```python
from build123d import *

# Parameters (mm, degrees)
F0_W      = 59
F0_H      = 54
F1_DEPTH  = 5
F2_W      = 5
F2_H      = 54
F3_DEPTH  = 21.25
F4_W      = 42
F4_H      = 42
F5_DEPTH  = 9.75
F7_DEPTH  = 33
F8_R      = 1.6
F8_R_2    = 11.5
F9_DEPTH  = 14.751
F10_R     = 2.1
F11_DEPTH = 5.001
F12_SIZE  = 3
F13_R     = 5
F14_R     = 1.6
F15_DEPTH = 2.5
F16_R     = 2.1
F17_DEPTH = 59.001
F19_DEPTH = 10.6937211186


with BuildPart() as f1:
    # F0 (on Top) → F1 (new body)
    with BuildSketch(Plane.XY):
        with Locations((29.5, 27)):
            Rectangle(F0_W, F0_H)
    extrude(amount=F1_DEPTH)

    # F2 (on face) → F3 (join)
    with BuildSketch(Plane.XY.offset(5)):
        with Locations((2.5, 27)):
            Rectangle(F2_W, F2_H)
    extrude(amount=F3_DEPTH)

    # F4 (on face) → F5 (join)
    with BuildSketch(Plane.XY.offset(5)):
        with Locations((38, 21)):
            Rectangle(F4_W, F4_H)
    extrude(amount=F5_DEPTH)

    # F6 (on face) → F7 (cut)
    with BuildSketch(Plane.YZ.offset(59)):
        Polygon((0, 6.5), (0, 0), (33, 0), (19, 6.5), align=None)
    extrude(amount=-F7_DEPTH, mode=Mode.SUBTRACT)

    # F8 (on face) → F9 (cut, through all)
    with BuildSketch(Plane.XY.offset(14.75)):
        with Locations((22.8, 36.2)):
            Circle(F8_R)
        with Locations((38, 21)):
            Circle(F8_R_2)
        with Locations((53.2, 36.2)):
            Circle(F8_R)
        with Locations((22.8, 5.8)):
            Circle(F8_R)
        with Locations((53.2, 5.8)):
            Circle(F8_R)
        with Locations((29.8, 5.8)):
            Circle(F8_R)
    extrude(amount=-F9_DEPTH, mode=Mode.SUBTRACT)

    # F10 (on face) → F11 (cut, through all)
    with BuildSketch(Plane.XY.offset(5)):
        with Locations((37, 48)):
            Circle(F10_R)
        with Locations((51.5, 48)):
            Circle(F10_R)
    extrude(amount=-F11_DEPTH, mode=Mode.SUBTRACT)

    # F12
    f12_edges = [f1.edges().sort_by_distance(p)[0] for p in [
        (59, 54, 2.5),
        (59, 42, 9.875),
        (59, 0, 10.625),
    ]]
    chamfer(f12_edges, length=F12_SIZE)

    # F13
    f13_edges = [f1.edges().sort_by_distance(p)[0] for p in [
        (0, 27, 0),
    ]]
    fillet(f13_edges, radius=F13_R)

    # F14 (on face) → F15 (cut)
    with BuildSketch(Plane.XY.offset(14.75)):
        Polygon((31.417729554, 3.0006632601), (33.0331615075, 5.8013265202), (31.4154319535, 8.6006632601), (28.182270446, 8.5993367399), (26.5668384925, 5.7986734798), (28.1845680465, 2.9993367399), align=None)
        with Locations((29.8, 5.8)):
            Circle(F14_R, mode=Mode.SUBTRACT)
    extrude(amount=-F15_DEPTH, mode=Mode.SUBTRACT)

    # F16 (on face) → F17 (cut, through all)
    with BuildSketch(Plane(origin=(0, 0, 0), x_dir=(0, -1, 0), z_dir=(-1, 0, 0))):
        with Locations((-36.9, 20)):
            Circle(F16_R)
        with Locations((-4.9, 20)):
            Circle(F16_R)
    extrude(amount=-F17_DEPTH, mode=Mode.SUBTRACT)

    # F18 (on face) → F19 (cut, through all)
    with BuildSketch(Plane.XZ):
        with BuildLine():
            Line((32.9, 9.5), (32.9, 6.5))
            Line((32.9, 6.5), (41.1, 6.5))
            Line((41.1, 6.5), (41.1, 9.5))
            ThreePointArc((41.1, 9.5), (37, 13.6), (32.9, 9.5))
        make_face()
    extrude(amount=-F19_DEPTH, mode=Mode.SUBTRACT)


solid = f1.part
```
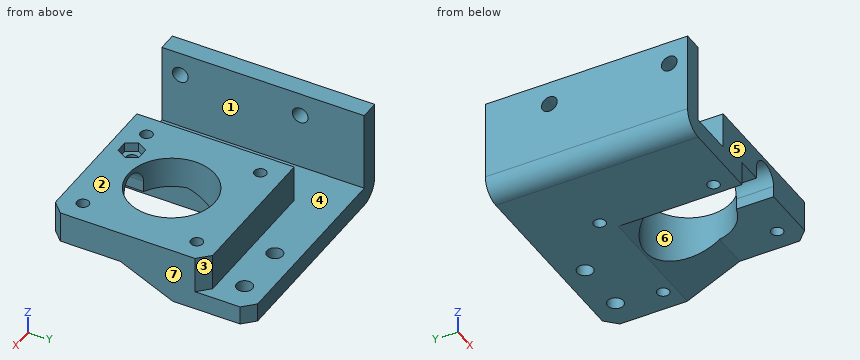
Geometry check sheet. Reference: the model listing, model coordinates, mm. Face numbers are marked on the shaded views. A direction names the side the tool comes from. Give positions to 0.01 mm unless a question says otherwise; leave off trailing zeros. Write each loop counter-clockwise with the first axis right and the second up, starting at its lowest first coordinate (ties: lowest second). Pieces come first, ordered by that corner, then holes. Notation, with made-up numbers: (-0.5, -7) - (44.5, -7) arc R18 cw to (44.5, 2) - close; hole circle Ø4 at (46, -33.75). An arc over 180 degrees is marked (long way). Use a Markdown table: item, result.
Q1. Section check B-B, the plane x = 22.8. Enter the section's corners in (y, z).
Computed:
| item | result |
|---|---|
| outline | (0, 0) - (4.2, 0) - (4.2, 14.75) - (0, 14.75) - close; (7.4, 0) - (34.6, 0) - (34.6, 14.75) - (7.4, 14.75) - close; (37.8, 0) - (54, 0) - (54, 5) - (42, 5) - (42, 14.75) - (37.8, 14.75) - close |
Q2. Section check A-A, the plane z = 8.5. Enter the section's corners in (x, y), then the cut area to 3 significant figures.
Computed:
| item | result |
|---|---|
| outline | (0, 0) - (5, 0) - (5, 54) - (0, 54) - close; (17, 0) - (32.9, 0) - (32.9, 10.69) arc R11.5 cw (long way) to (41.1, 9.93) - (41.1, 0) - (56, 0) - (59, 3) - (59, 39) - (56, 42) - (17, 42) - close; hole circle Ø3.2 at (22.8, 5.8); hole circle Ø3.2 at (22.8, 36.2); hole circle Ø3.2 at (29.8, 5.8); hole circle Ø3.2 at (53.2, 5.8); hole circle Ø3.2 at (53.2, 36.2) |
| area | 1,490 mm² |
Q3. Section check C-C, the plane y = 13. Enter the section's corners in (x, z).
Computed:
| item | result |
|---|---|
| outline | (0, 5) arc R5 ccw to (5, 0) - (26, 0) - (26, 6.5) - (29.74, 6.5) - (29.74, 14.75) - (17, 14.75) - (17, 5) - (5, 5) - (5, 26.25) - (0, 26.25) - close; (46.26, 6.5) - (59, 6.5) - (59, 14.75) - (46.26, 14.75) - close |
Q4. Go/stop test with flat-tipped pins: P1, Ø5, axis at x = 29.8, y = 5.8, coming from the -Z side; P2, Ø2, axis at x = 34.5, y = 7.5, coming from the -Z side; P3, Ø14.5, axis at x = 48, y = 13, coming from the -Z side. Record where each tip stops, or that it passes through.
Computed:
| item | result |
|---|---|
| P1 | stops at z = 6.5 |
| P2 | stops at z = 11.64 |
| P3 | stops at z = 5.99 |
Q5. Section check D-D, the plane y = 36.2. Enter the section's corners in (x, z).
Computed:
| item | result |
|---|---|
| outline | (0, 5) arc R5 ccw to (5, 0) - (21.2, 0) - (21.2, 14.75) - (17, 14.75) - (17, 5) - (5, 5) - (5, 18.02) - (0, 18.02) - close; (0, 21.98) - (5, 21.98) - (5, 26.25) - (0, 26.25) - close; (24.4, 0) - (51.6, 0) - (51.6, 14.75) - (24.4, 14.75) - close; (54.8, 0) - (59, 0) - (59, 14.75) - (54.8, 14.75) - close |
Q6. Set-up check for the marked faces 1, 2, 3 and 4: record each of +Z, -Z, +X, -X, +Y, -Y from which the full face is reachable in a straight line by a thin tool's end or side.
Computed:
| item | result |
|---|---|
| face 1 | +Z, +Y, -Y |
| face 2 | +Z, +X, +Y, -Y |
| face 3 | +Z, +X, +Y |
| face 4 | +Z, +Y |
Q7. Draft check along X on the marked faces 5, 6 and 7. Enter one of: pulls with the +X half, pulls with the -X half, needs draft (parallel to the pull), parting line crosses it, or undercut.
Computed:
| item | result |
|---|---|
| face 5 | needs draft |
| face 6 | undercut |
| face 7 | pulls with the +X half |
Q8. Thickness scan on L1, parallel to Y at x = 22.8, z = 4.25; L2, parallel to X at y = 28.5, z = 13.75; L3, parallel to Z at x = 18.5, y = 39.5. Record the ranges inside material, lowest first. Write a range as [from, to].
Computed:
| item | result |
|---|---|
| L1 | y = [0, 4.2], [7.4, 34.6], [37.8, 54] |
| L2 | x = [0, 5], [17, 29.28], [46.72, 59] |
| L3 | z = [0, 14.75] |
